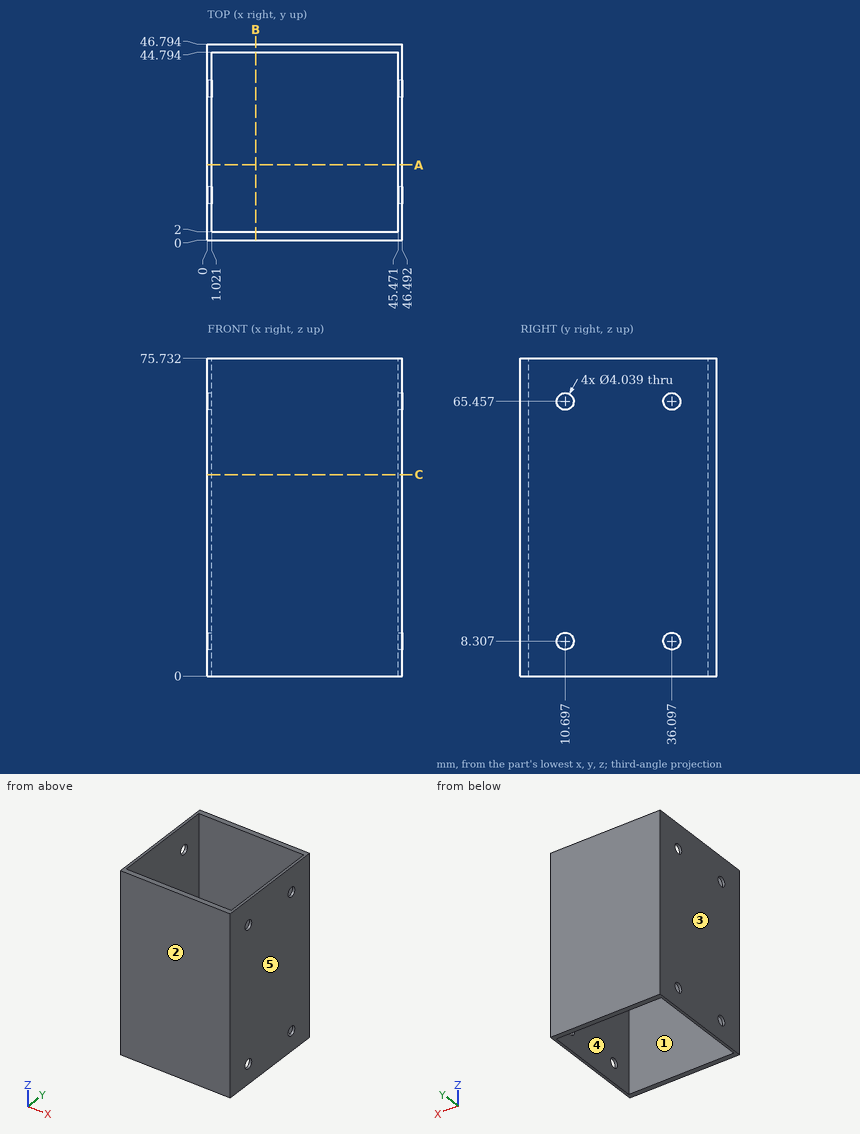
Source: three-view drawing plus pictorial views. Frame: mm from the lowest corner of the part. A direction names the side the tool comes from. Give positions to 0.01 mm unless a question says otherwise; leave off trailing zeros. Write each loop counter-clockwise with the first axis right and the second up, starting at its lowest first coordinate (ties: lowest second). Pieces come first, ordered by that corner, then holes. Notation, with made-up numbers: (-20.75, -17) -> (-14.75, -17) arc R21 cw to (-14.75, -1) -> close; hole circle Ø3 at (-28.5, 36). An arc over 180 degrees is marked (long way). Answer in a Markdown table with one row per item.
(1) Draft query along Y for the marked faces 1, 2 and 3. Return one class per face: +Y half, -Y half, draft (parallel to the pull), parting line (faces both ways), or undercut.
Answers below:
| item | result |
|---|---|
| face 1 | undercut |
| face 2 | -Y half |
| face 3 | draft |
(2) Section query C-C on z = 48. Return loops of the section in (x, y) (1 decimal).
Answers below:
| item | result |
|---|---|
| outline | (0, 0) -> (46.5, 0) -> (46.5, 46.8) -> (0, 46.8) -> close; hole (1, 2) -> (45.5, 2) -> (45.5, 44.8) -> (1, 44.8) -> close |
(3) Pin query (flat end, axial travel): pin 1 (2.5 mm diameter, centred on y = 10.7, z = 8.31, fed in from -X). Return the tip coordinate at first contact, or that it passes through.
Answers below:
| item | result |
|---|---|
| pin 1 | through |
(4) Set-up query: the marked faces 4 and 5. Return all of +Z, -Z, +X, -X, +Y, -Y with unobstructed straight access to the full face (end or side cutting, diameter ignored); none if empty.
Answers below:
| item | result |
|---|---|
| face 4 | +Z, -Z |
| face 5 | +Z, -Z, +X, +Y, -Y |
(5) Section query B-B on x = 11.5. Return loops of the section in (y, z) (1 decimal).
Answers below:
| item | result |
|---|---|
| outline | (0, 0) -> (2, 0) -> (2, 75.7) -> (0, 75.7) -> close; (44.8, 0) -> (46.8, 0) -> (46.8, 75.7) -> (44.8, 75.7) -> close |
(6) Ray query, line 1 along Y through (x, z) = (26.5, 24) (1 decimal); line 2 along X through (y, z) = (42.5, 5.5). Return the intervals inside material, ascending. Write a range as [from, to].
Answers below:
| item | result |
|---|---|
| line 1 | [0, 2], [44.8, 46.8] |
| line 2 | [0, 1.02], [45.47, 46.49] |
(7) Section query A-A on y = 18. Return loops of the section in (x, z).
Answers below:
| item | result |
|---|---|
| outline | (0, 0) -> (1.02, 0) -> (1.02, 75.73) -> (0, 75.73) -> close; (45.47, 0) -> (46.49, 0) -> (46.49, 75.73) -> (45.47, 75.73) -> close |
